from build123d import *

# Parameters (mm, degrees)
SKETCH_2_R          = 7.5
SKETCH_2_R_2        = 3.65
EXTRUDE_1_DEPTH     = 4
SKETCH_3_W          = 65
SKETCH_3_H          = 34.5
SKETCH_3_R          = 3.65
EXTRUDE_2_DEPTH     = 2
EXTRUDE_3_DEPTH     = 4
SKETCH_5_W          = 10
SKETCH_5_H          = 2
CUT_EXTRUDE_1_DEPTH = 3.7
FILLET_1_R          = 1.5
SKETCH_6_W          = 2
SKETCH_6_H          = 10
CUT_EXTRUDE_2_DEPTH = 5
SKETCH_7_W          = 1
SKETCH_7_H          = 10
CUT_EXTRUDE_3_DEPTH = 5.5


with BuildPart() as part:
    # 草图2 → 凸台-拉伸1 (new body)
    with BuildSketch(Plane.XY):
        Circle(SKETCH_2_R)
        Circle(SKETCH_2_R_2, mode=Mode.SUBTRACT)
    extrude(amount=EXTRUDE_1_DEPTH)

    # 草图3 → 凸台-拉伸2 (add)
    with BuildSketch(Plane.XY.offset(4)):
        with Locations((-2.5, -7.75)):
            Rectangle(SKETCH_3_W, SKETCH_3_H)
        Circle(SKETCH_3_R, mode=Mode.SUBTRACT)
    extrude(amount=EXTRUDE_2_DEPTH)

    # 草图4 → 凸台-拉伸3 (add)
    with BuildSketch(Plane(origin=(0, 0, 4), x_dir=(-1, 0, 0), z_dir=(0, 0, -1))):
        Polygon((-28, 7.5), (-28, -23), (33, -23), (33, 7.5), (33, 9.5), (35, 9.5), (35, -25), (-30, -25), (-30, 9.5), (-28, 9.5), align=None)
    extrude(amount=EXTRUDE_3_DEPTH)

    # 草图5 → 切除-拉伸1 (cut)
    with BuildSketch(Plane(origin=(0, 0, 0), x_dir=(-1, 0, 0), z_dir=(0, 0, -1))):
        with Locations((0, -24)):
            Rectangle(SKETCH_5_W, SKETCH_5_H)
    extrude(amount=-CUT_EXTRUDE_1_DEPTH, mode=Mode.SUBTRACT)

    # 圆角1
    fillet_1_edges = [part.edges().sort_by_distance(p)[0] for p in [
        (5, -24, 3.7),
        (-5, -24, 3.7),
    ]]
    fillet(fillet_1_edges, radius=FILLET_1_R)

    # 草图6 → 切除-拉伸2 (cut)
    with BuildSketch(Plane(origin=(0, 0, 0), x_dir=(-1, 0, 0), z_dir=(0, 0, -1))):
        with Locations((34, -2)):
            Rectangle(SKETCH_6_W, SKETCH_6_H)
    extrude(amount=-CUT_EXTRUDE_2_DEPTH, mode=Mode.SUBTRACT)

    # 草图7 → 切除-拉伸3 (cut)
    with BuildSketch(Plane.ZY.offset(33)):
        with Locations((4.5, -2)):
            Rectangle(SKETCH_7_W, SKETCH_7_H)
    extrude(amount=-CUT_EXTRUDE_3_DEPTH, mode=Mode.SUBTRACT)


solid = part.part
Verification items for the finished model (mm, model axes). A direction names the side the tool comes from. Give positions to 0.01 mm unless a question says otherwise; leave off trailing zeros. Write each loop counter-clockwise with the first axis right and the second up, starting at its lowest first coordinate (ties: lowest second). Pieces come first, ordered by that corner, then holes.
(1) Cross-section at A-A (x = 0). Enter the section's corners in (y, z), plus the area to 3 significant figures.
(2) Cross-section at B-B (y = -20). Enter the section's corners in (x, z), plus the area to 3 significant figures.
(3) Mould release check, pull along X, two halves, no side actions. Record for faces 4 (the face through (28, -7, 2)), 5 (the face through (-35, -8, 3)), 6 (the face through (30, -8, 3)), 7 (the face through (-34, -7, 4)): +X half, -X half, draft (parallel to the pull), parting line (faces both ways), or undercut.
(4) Gauge pin test, flat ends, axial feed: pin 1 (0.6 mm diameter, centred on x = 1.5, y = -23.5, fed in from -Z); pin 2 (5 mm diameter, centred on x = 2, y = -20, fed in from -Z); pin 3 (2 mm diameter, centred on x = 13.5, z = 1, fed in from +Y). Record the tip position at first contact, or that the pin passes through.
(5) Material ranges on line 1 (X direction, y = -16, z = 2.5); line 2 (Z direction, x = 18, y = -5); line 3 (Y direction, x = 0, z = 3.6), recorded low to high.
(6) Access from +Z, -Z, +X, -X, +Y, -Y to the whole of each face (thin tool, end or side, straight path). Record for faces 1 (the face through (-33, 6, 2)), 2 (the face through (-5, -24, 1)), 3 (the face through (-3, -10, 4)).
(7) Cross-section at D-D (x = -10). Enter the section's corners in (y, z), plus the area to 3 significant figures.
(8) Cross-section at C-C (y = 0). Enter the section's corners in (x, z), plus the area to 3 significant figures.
Worked out:
1. outline: (-25, 3.7) - (-23, 3.7) - (-23, 4) - (-7.5, 4) - (-7.5, 0) - (-3.65, 0) - (-3.65, 6) - (-25, 6) - close; (3.65, 0) - (7.5, 0) - (7.5, 4) - (9.5, 4) - (9.5, 6) - (3.65, 6) - close
1. area: 85.8 mm2
2. outline: (-35, 0) - (-33, 0) - (-33, 4) - (28, 4) - (28, 0) - (30, 0) - (30, 6) - (-35, 6) - close
2. area: 146 mm2
3. face 4: undercut
3. face 5: -X half
3. face 6: +X half
3. face 7: draft
4. pin 1: stops at z = 3.7
4. pin 2: stops at z = 4
4. pin 3: stops at y = -23
5. line 1: x = -35 to -33, 28 to 30
5. line 2: z = 4 to 6
5. line 3: y = -7.5 to -3.65, 3.65 to 7.5
6. face 1: -Z, +Y
6. face 2: -Z, -Y
6. face 3: -Z
7. outline: (-25, 0) - (-23, 0) - (-23, 4) - (9.5, 4) - (9.5, 6) - (-25, 6) - close
7. area: 77.0 mm2
8. outline: (-35, 5) - (-27.5, 5) - (-27.5, 4) - (-7.5, 4) - (-7.5, 0) - (-3.65, 0) - (-3.65, 6) - (-35, 6) - close; (3.65, 0) - (7.5, 0) - (7.5, 4) - (28, 4) - (28, 0) - (30, 0) - (30, 6) - (3.65, 6) - close
8. area: 147 mm2
